The model under review builds one solid part; all positions refer to its coordinate system, in mm. Face numbers are marked on the shaded views. A direction names the side the tool comes from. Coordinates: 2 decimals unless noted, no trailing zeros. Order: outer loops, then holes, each group sorted by start corner. A loop starts at its lowest first (then second) coordinate and runs counter-clockwise, first axis right, second up. Notation, with made-up numbers: M -33.5,71.25 L 15.5,71.25 A24 cw 15.5,89.25 Z; hole C 47,24 d9. An arc over 180 degrees is marked long. Answer in a Markdown table with one row per item.
from build123d import *

# Parameters (mm, degrees)
SKETCH1_W           = 25
SKETCH1_H           = 28.2
BOSS_EXTRUDE1_DEPTH = 2
BOSS_EXTRUDE2_DEPTH = 5
LPATTERN1_COUNT     = 3
LPATTERN1_PITCH     = 10
SKETCH6_R           = 1.050000034
CUT_EXTRUDE1_DEPTH  = 31.490326335
FILLET1_R           = 1
FILLET2_R           = 1


with BuildPart() as part:
    # Sketch1 → Boss-Extrude1 (new body)
    with BuildSketch(Plane.XY):
        Rectangle(SKETCH1_W, SKETCH1_H)
    extrude(amount=BOSS_EXTRUDE1_DEPTH)

    # Sketch5 → Boss-Extrude2 (add)
    with BuildSketch(Plane.ZY.offset(12.5)):
        with BuildLine():
            Line((0.5, 15.6), (0, 14.1))
            Line((0, 14.1), (2, 14.1))
            ThreePointArc((2, 14.1), (3.060660172, 16.660660172), (0.5, 15.6))
        make_face()
    boss_extrude2 = extrude(amount=-BOSS_EXTRUDE2_DEPTH)

    # LPattern1: Boss-Extrude2 ×3
    with Locations(*[(i * LPATTERN1_PITCH, 0, 0) for i in range(1, LPATTERN1_COUNT)]):
        add(boss_extrude2)

    # Sketch6 → Cut-Extrude1 (cut, through all)
    with BuildSketch(Plane.ZY.offset(12.5)):
        with Locations((2, 15.6)):
            Circle(SKETCH6_R)
    extrude(amount=-CUT_EXTRUDE1_DEPTH, mode=Mode.SUBTRACT)

    # Fillet1
    # the kernel refuses this fillet: 1 mm, written as the material it takes off along each edge
    with BuildSketch(Plane(origin=(12.5, -20.1, 0), x_dir=(0, 0, 1), z_dir=(0, 1, 0)), Plane(origin=(-12.5, 20.1, 0), x_dir=(0, 0, 1), z_dir=(0, -1, 0))) as fillet1_piece_1:
        with BuildLine():
            CenterArc((FILLET1_R, -FILLET1_R), FILLET1_R, 90, 90)
            Line((0, -FILLET1_R), (-FILLET1_R * 0.02, -FILLET1_R))
            Line((-FILLET1_R * 0.02, -FILLET1_R), (-FILLET1_R * 0.02, FILLET1_R * 0.02))
            Line((-FILLET1_R * 0.02, FILLET1_R * 0.02), (FILLET1_R, FILLET1_R * 0.02))
            Line((FILLET1_R, FILLET1_R * 0.02), (FILLET1_R, 0))
        make_face()
    extrude(amount=40.2, mode=Mode.SUBTRACT)
    with BuildSketch(Plane(origin=(-18.5, -14.1, 0), x_dir=(0, 0, 1), z_dir=(1, 0, 0))) as fillet1_piece_2:
        with BuildLine():
            CenterArc((FILLET1_R, -FILLET1_R), FILLET1_R, 90, 90)
            Line((0, -FILLET1_R), (-FILLET1_R * 0.02, -FILLET1_R))
            Line((-FILLET1_R * 0.02, -FILLET1_R), (-FILLET1_R * 0.02, FILLET1_R * 0.02))
            Line((-FILLET1_R * 0.02, FILLET1_R * 0.02), (FILLET1_R, FILLET1_R * 0.02))
            Line((FILLET1_R, FILLET1_R * 0.02), (FILLET1_R, 0))
        make_face()
    extrude(amount=37, mode=Mode.SUBTRACT)

    # Fillet2
    # the kernel refuses this fillet: 1 mm, written as the material it takes off along each edge
    with BuildSketch(Plane(origin=(-11.5, -13.1, 1), x_dir=(-1, 0, 0), z_dir=(0, -1, 0))) as fillet2_piece_1_section:
        Polygon((0, 0), (FILLET2_R, 0), (FILLET2_R, FILLET2_R), (0, FILLET2_R), align=None)
    fillet2_piece_1 = extrude(amount=FILLET2_R, mode=Mode.PRIVATE)
    fillet2_piece_1 = fillet2_piece_1 - Plane(origin=(-11.5, -13.1, 1), x_dir=(0.7071067811865475, 0, 0.7071067811865475), z_dir=(0, -1, 0)) * Sphere(FILLET2_R, mode=Mode.PRIVATE)
    add(fillet2_piece_1, mode=Mode.SUBTRACT)
    with BuildSketch(Plane(origin=(11.5, -13.1, 1), x_dir=(1, 0, 0), z_dir=(0, -1, 0))) as fillet2_piece_2_section:
        Polygon((0, 0), (FILLET2_R, 0), (FILLET2_R, -FILLET2_R), (0, -FILLET2_R), align=None)
    fillet2_piece_2 = extrude(amount=FILLET2_R, mode=Mode.PRIVATE)
    fillet2_piece_2 = fillet2_piece_2 - Plane(origin=(11.5, -13.1, 1), x_dir=(-0.7071067811865475, 0, 0.7071067811865475), z_dir=(0, -1, 0)) * Sphere(FILLET2_R, mode=Mode.PRIVATE)
    add(fillet2_piece_2, mode=Mode.SUBTRACT)
    with BuildSketch(Plane(origin=(12.5, -14.1, 1), x_dir=(-1, 0, 0), z_dir=(0, 0, 1))) as fillet2_piece_3:
        with BuildLine():
            CenterArc((FILLET2_R, -FILLET2_R), FILLET2_R, 90, 90)
            Line((0, -FILLET2_R), (0, 0))
            Line((0, 0), (FILLET2_R, 0))
        make_face()
    extrude(amount=3.5, mode=Mode.SUBTRACT)
    with BuildSketch(Plane(origin=(-12.5, -14.1, 1), x_dir=(1, 0, 0), z_dir=(0, 0, 1))) as fillet2_piece_4:
        with BuildLine():
            CenterArc((FILLET2_R, FILLET2_R), FILLET2_R, 180, 90)
            Line((0, FILLET2_R), (0, 0))
            Line((0, 0), (FILLET2_R, 0))
        make_face()
    extrude(amount=3.5, mode=Mode.SUBTRACT)


solid = part.part
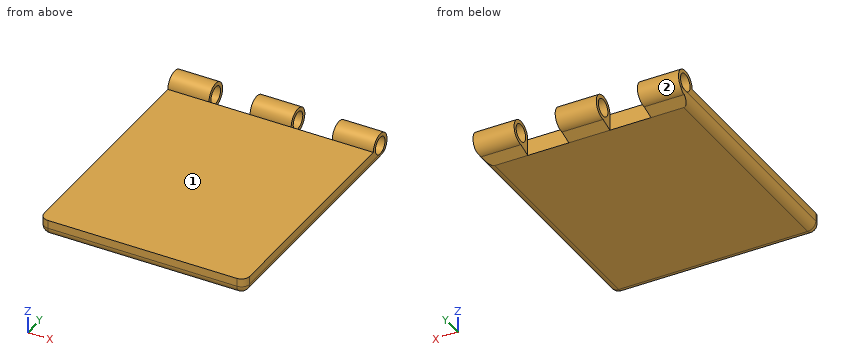
(1) Take a section at B-B (y = -10). Write out the cut boundary in (x, z), then the cut area to 3 significant figures.
Report:
| item | result |
|---|---|
| outline | M -12.5,1 A1 ccw -11.5,0 L 11.5,0 A1 ccw 12.5,1 L 12.5,2 L -12.5,2 Z |
| area | 49.6 mm^2 |
(2) Machinability: for the marked faces 1 and 2, which of the approach directions +Z, -Z, +X, -X, +Y, -Y give a long, thin tool a straight path to every point of the face, cutting with its end or side? Answer none if there is none.
Report:
| item | result |
|---|---|
| face 1 | +Z, +X, -X, -Y |
| face 2 | +X, -X |
(3) To check wall thickness, follow line 1 (X direction, y = 14.5, z = 1.95); line 2 (Y direction, x = 10.5, z = 1.9); line 3 (Z direction, x = -9.75, y = -11.5). State the ranges of each line that lie inside material, in increasing order. Write a range as [from, to].
Report:
| item | result |
|---|---|
| line 1 | [-12.5, -7.5], [-2.5, 2.5], [7.5, 12.5] |
| line 2 | [-14.1, 14.55], [16.65, 17.1] |
| line 3 | [0, 2] |
(4) Take a section at A-A (x = -8). Write out the cut boundary in (y, z).
Report:
| item | result |
|---|---|
| outline | M -14.1,1 A1 ccw -13.1,0 L 14.1,0 L 15.6,0.5 A1.5 ccw long 14.1,2 L -14.1,2 Z; hole C 15.6,2 d2.1 |
(5) Insertion check: P1, Ø1.6, axis at x = 4, z = 1, coming from the +Y side; P2, Ø8, axis at x = -6.5, y = -3.5, coming from the +Z side. Each pin has a flat end and moves straight along its axis. Give the tip position at first contact, or say it passes through.
Report:
| item | result |
|---|---|
| P1 | y = 14.1 |
| P2 | z = 2 |
(6) Take a section at C-C (x = -3.5). Write out the cut boundary in (y, z), then the cut area to 3 significant figures.
Report:
| item | result |
|---|---|
| outline | M -14.1,1 A1 ccw -13.1,0 L 14.1,0 L 14.1,2 L -14.1,2 Z |
| area | 56.2 mm^2 |
